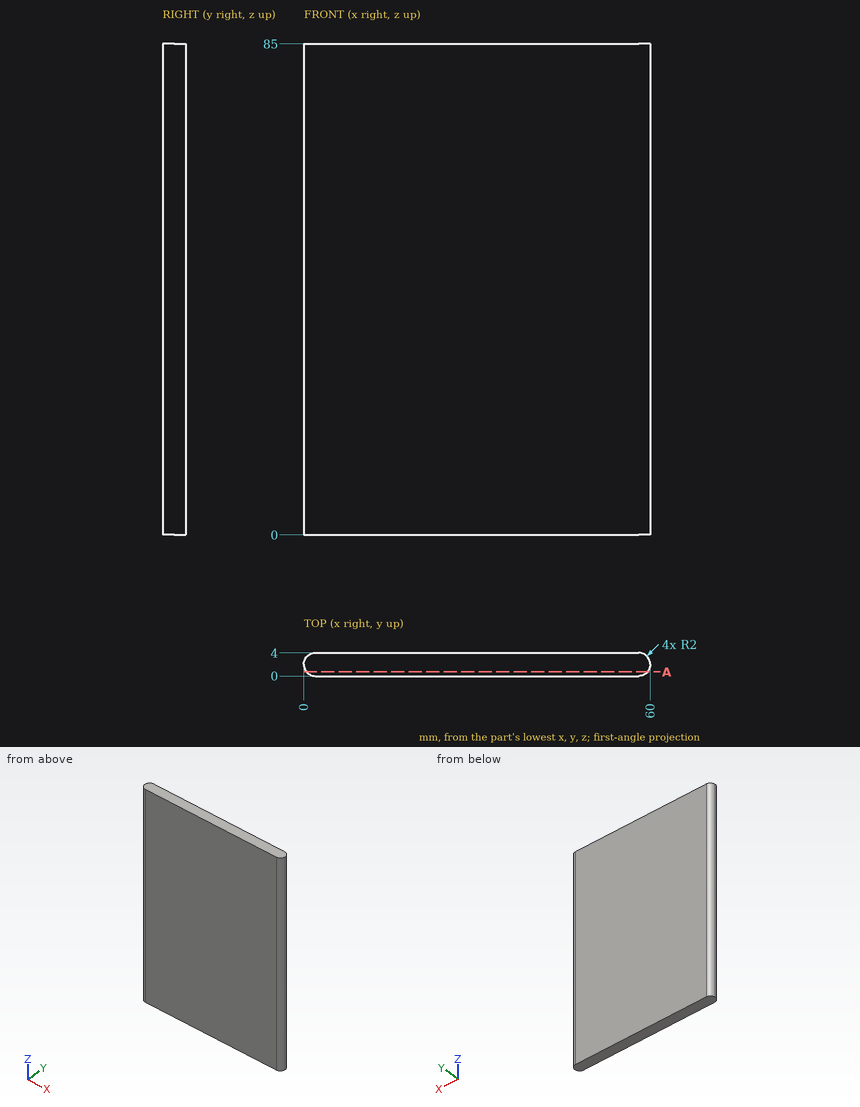
Study the drawing (mm; zero at the part's minimum x, y, z) and answer. Give positions to 0.01 mm unless a question says otherwise; leave off trailing zeros. Write each loop counter-clockwise with the first axis right and the second up, starting at its lowest first coordinate (ties: lowest second). Pieces come first, ordered by that corner, then holes. Notation, with made-up numbers: (18.5, 59) - (55.5, 59) arc R18 ccw to (55.5, 75) - close; hole circle Ø11 at (-39, 64). An arc over 180 degrees is marked (long way). Write item = value, one per line. Start each with the question number.
Item 1: Find the intervals of material crossed by probe 1 along X at (y, z) = (1.8, 13); probe 2 along X at (y, z) = (0.6, 33), in increasing order. Write a range as [from, to].
Item 2: This flat-tipped pin is pushed along its axis until it touches: P1, Ø2, axis at x = 28.5, y = 0.5, coming from the -Z side. Where does it stop, or does it pass through?
Item 3: Find section A-A (y = 0.7). Give the vertices of the cut face in (x, z), then the cut area to 3 significant figures.
Response:
q1.probe_1 = [0.01, 59.99]
q1.probe_2 = [0.57, 59.43]
q2.P1 = 0
q3.outline = (0.48, 0) - (59.52, 0) - (59.52, 85) - (0.48, 85) - close
q3.area = 5,020 mm²
